from build123d import *
from build123d.topology import SkipClean

# Parameters (mm, degrees)
F_4_40_TAPPED_HOLE1_D               = 2.2606
F_4_40_TAPPED_HOLE1_DEPTH           = 7.62
F_4_40_TAPPED_HOLE1_TIP             = 0.679152758
F_4_40_TAPPED_HOLE1_ON_FACE_2_D     = 2.2606
F_4_40_TAPPED_HOLE1_ON_FACE_2_DEPTH = 7.62
F_4_40_TAPPED_HOLE1_ON_FACE_2_TIP   = 0.679152758
F_4_40_TAPPED_HOLE1_ON_FACE_3_D     = 2.2606
F_4_40_TAPPED_HOLE1_ON_FACE_3_DEPTH = 7.62
F_4_40_TAPPED_HOLE1_ON_FACE_3_TIP   = 0.679152758
F_4_40_TAPPED_HOLE1_ON_FACE_4_D     = 2.2606
F_4_40_TAPPED_HOLE1_ON_FACE_4_DEPTH = 7.62
F_4_40_TAPPED_HOLE1_ON_FACE_4_TIP   = 0.679152758
SKETCH10_R                          = 20.50415
CUT_EXTRUDE3_DEPTH                  = 31.75
F_4_40_TAPPED_HOLE2_D               = 2.2606
F_4_40_TAPPED_HOLE2_DEPTH           = 7.62
F_4_40_TAPPED_HOLE2_TIP             = 0.679152758
CHAMFER1_SIZE                       = 1.27
SKETCH23_R                          = 26.9621
CUT_EXTRUDE6_DEPTH                  = 10
CUT_EXTRUDE7_DEPTH                  = 21.75
FILLET2_R                           = 3.556


# Read off the part's stored shape, not the designer's step: AdvancedHole3
with BuildPart() as part:
    # Sketch2 → Revolve1 (revolve)
    with BuildSketch(Plane(origin=(0, 0, 0), x_dir=(0, 0, -1), z_dir=(1, 0, 0))):
        Polygon((-18.542, 30.02915), (-12.192, 30.02915), (-12.192, 27.9781), (-8.5725, 27.9781), (-8.5725, 30.02915), (-6.0325, 30.02915), (-6.0325, 27.9781), (-2.413, 27.9781), (-2.413, 30.02915), (0, 30.02915), (0, 0), (-18.542, 0), align=None)
    revolve(axis=Axis((0, 0, 0), (0, 0, 1)))

    # #4-40 Tapped Hole1
    with Locations(Plane(origin=(0, -30.02915, 15.367), x_dir=(0, 0, -1), z_dir=(0, -1, 0))):
        with Locations((0, 0)):
            Hole(F_4_40_TAPPED_HOLE1_D / 2, depth=F_4_40_TAPPED_HOLE1_DEPTH)
            with Locations((0, 0, -(F_4_40_TAPPED_HOLE1_DEPTH + F_4_40_TAPPED_HOLE1_TIP / 2))):  # 118° drill point
                Cone(0, F_4_40_TAPPED_HOLE1_D / 2, F_4_40_TAPPED_HOLE1_TIP, mode=Mode.SUBTRACT)

    # #4-40 Tapped Hole1 on face 2
    with Locations(Plane(origin=(30.02915, 0, 15.367), x_dir=(0, 0, 1), z_dir=(1, 0, 0))):
        with Locations((0, 0)):
            Hole(F_4_40_TAPPED_HOLE1_ON_FACE_2_D / 2, depth=F_4_40_TAPPED_HOLE1_ON_FACE_2_DEPTH)
            with Locations((0, 0, -(F_4_40_TAPPED_HOLE1_ON_FACE_2_DEPTH + F_4_40_TAPPED_HOLE1_ON_FACE_2_TIP / 2))):  # 118° drill point
                Cone(0, F_4_40_TAPPED_HOLE1_ON_FACE_2_D / 2, F_4_40_TAPPED_HOLE1_ON_FACE_2_TIP, mode=Mode.SUBTRACT)

    # #4-40 Tapped Hole1 on face 3
    with Locations(Plane(origin=(-30.02915, 0, 15.367), x_dir=(0, 0, -1), z_dir=(-1, 0, 0))):
        with Locations((0, 0)):
            Hole(F_4_40_TAPPED_HOLE1_ON_FACE_3_D / 2, depth=F_4_40_TAPPED_HOLE1_ON_FACE_3_DEPTH)
            with Locations((0, 0, -(F_4_40_TAPPED_HOLE1_ON_FACE_3_DEPTH + F_4_40_TAPPED_HOLE1_ON_FACE_3_TIP / 2))):  # 118° drill point
                Cone(0, F_4_40_TAPPED_HOLE1_ON_FACE_3_D / 2, F_4_40_TAPPED_HOLE1_ON_FACE_3_TIP, mode=Mode.SUBTRACT)

    # #4-40 Tapped Hole1 on face 4
    with Locations(Plane(origin=(0, 30.02915, 15.367), x_dir=(0, 0, 1), z_dir=(0, 1, 0))):
        with Locations((0, 0)):
            Hole(F_4_40_TAPPED_HOLE1_ON_FACE_4_D / 2, depth=F_4_40_TAPPED_HOLE1_ON_FACE_4_DEPTH)
            with Locations((0, 0, -(F_4_40_TAPPED_HOLE1_ON_FACE_4_DEPTH + F_4_40_TAPPED_HOLE1_ON_FACE_4_TIP / 2))):  # 118° drill point
                Cone(0, F_4_40_TAPPED_HOLE1_ON_FACE_4_D / 2, F_4_40_TAPPED_HOLE1_ON_FACE_4_TIP, mode=Mode.SUBTRACT)

    # Sketch6 → Revolve2 (revolve)
    with BuildSketch(Plane(origin=(0, 0, 0), x_dir=(1, 0, 0), z_dir=(0, 1, 0)), mode=Mode.PRIVATE) as revolve2_sk:
        with BuildLine():
            Line((0, -18.542), (31.75, -18.542))
            ThreePointArc((31.75, -18.542), (22.450640303, -40.992640303), (0, -50.292))
            Line((0, -50.292), (0, -18.542))
        make_face()
    revolve(revolve2_sk.sketch.rotate(Axis((0, 0, 18.542), (0, 0, 1)), 90), axis=Axis((0, 0, 18.542), (0, 0, 1)))

    # Sketch10 → Cut-Extrude3 (cut)
    with BuildSketch(Plane(origin=(0, 0, 0), x_dir=(-1, 0, 0), z_dir=(0, 0, -1))):
        with Locations(Location((0, 0, 0), (0, 0, 90))):
            Circle(SKETCH10_R)
    extrude(amount=-CUT_EXTRUDE3_DEPTH, mode=Mode.SUBTRACT)

    # #4-40 Tapped Hole2
    with Locations(Plane(origin=(0, 0, 31.75), x_dir=(-1, 0, 0), z_dir=(0, 0, -1))):
        with Locations((0, 0)):
            Hole(F_4_40_TAPPED_HOLE2_D / 2, depth=F_4_40_TAPPED_HOLE2_DEPTH)
            with Locations((0, 0, -(F_4_40_TAPPED_HOLE2_DEPTH + F_4_40_TAPPED_HOLE2_TIP / 2))):  # 118° drill point
                Cone(0, F_4_40_TAPPED_HOLE2_D / 2, F_4_40_TAPPED_HOLE2_TIP, mode=Mode.SUBTRACT)

    # Chamfer1
    chamfer1_edges = [part.edges().sort_by_distance(p)[0] for p in [
        (0, -30.02915, 0),
    ]]
    chamfer(chamfer1_edges, length=CHAMFER1_SIZE)

    # AdvancedHole3 outline → AdvancedHole3 (revolve, cut)
    with BuildSketch(Plane.YX.offset(-36.83)):
        Polygon((3.81, 28.256858344), (0, 28.256858344), (0, 8.880183098), (2.5527, 10.414), (2.5527, 23.114), (3.81, 23.114), align=None)
    advancedhole3 = revolve(axis=Axis((0, 0, 36.83), (1, 0, 0)), mode=Mode.SUBTRACT)

    # Mirror2: AdvancedHole3 across plane
    add(advancedhole3.mirror(Plane(origin=(0, 0, 0), x_dir=(0, 0, 1), z_dir=(1, 0, 0))), mode=Mode.SUBTRACT)

    # Sketch23 → Cut-Extrude6 (cut)
    with BuildSketch(Plane(origin=(0, 0, 0), x_dir=(-1, 0, 0), z_dir=(0, 0, -1))):
        with Locations(Location((0, 0, 0), (0, 0, 90))):
            Circle(SKETCH23_R)
    extrude(amount=-CUT_EXTRUDE6_DEPTH, mode=Mode.SUBTRACT)

    # Sketch24 → Cut-Extrude7 (cut)
    with SkipClean():  # the faces are left unmerged after this step: merging them gives an invalid solid
        with BuildSketch(Plane(origin=(0, 0, 10), x_dir=(-1, 0, 0), z_dir=(0, 0, -1))):
            with BuildLine():
                Line((-5.972908248, 26.29218902), (-2.54, 20.346217516))
                Line((-2.54, 20.346217516), (2.54, 20.346217516))
                Line((2.54, 20.346217516), (5.972908248, 26.29218902))
                ThreePointArc((5.972908248, 26.29218902), (19.065083745, 19.065083745), (26.29218902, 5.972908248))
                Line((26.29218902, 5.972908248), (20.346217516, 2.54))
                Line((20.346217516, 2.54), (20.346217516, -2.54))
                Line((20.346217516, -2.54), (26.29218902, -5.972908248))
                ThreePointArc((26.29218902, -5.972908248), (19.065083745, -19.065083745), (5.972908248, -26.29218902))
                Line((5.972908248, -26.29218902), (2.54, -20.346217516))
                Line((2.54, -20.346217516), (-2.54, -20.346217516))
                Line((-2.54, -20.346217516), (-5.972908248, -26.29218902))
                ThreePointArc((-5.972908248, -26.29218902), (-19.065083745, -19.065083745), (-26.29218902, -5.972908248))
                Line((-26.29218902, -5.972908248), (-20.346217516, -2.54))
                Line((-20.346217516, -2.54), (-20.346217516, 2.54))
                Line((-20.346217516, 2.54), (-26.29218902, 5.972908248))
                ThreePointArc((-26.29218902, 5.972908248), (-19.065083745, 19.065083745), (-5.972908248, 26.29218902))
            make_face()
        extrude(amount=-CUT_EXTRUDE7_DEPTH, mode=Mode.SUBTRACT)

    # Fillet2
    fillet2_edges = [part.edges().sort_by_distance(p)[0] for p in [
        (26.29218902, 5.972908248, 20.875),
        (5.972908248, 26.29218902, 20.875),
        (-5.972908248, 26.29218902, 20.875),
        (-26.29218902, 5.972908248, 20.875),
        (-26.29218902, -5.972908248, 20.875),
        (-5.972908248, -26.29218902, 20.875),
        (5.972908248, -26.29218902, 20.875),
        (26.29218902, -5.972908248, 20.875),
    ]]
    fillet(fillet2_edges, radius=FILLET2_R)


solid = part.part
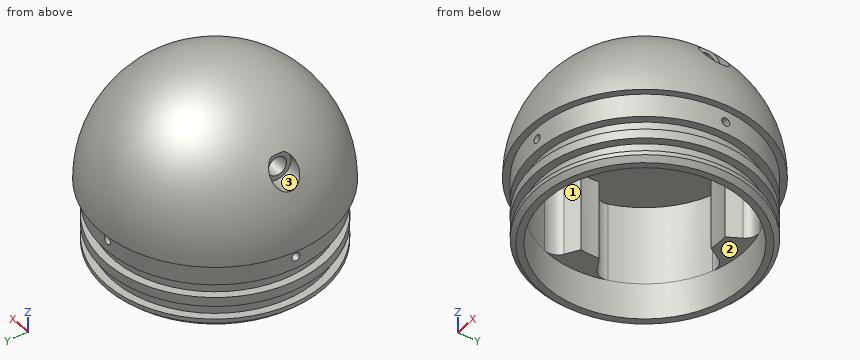
Source: CAD feature listing. Evaluate the final solid. Frame: model axes, mm. Face numbers are marked on the shaded views. Coordinates: 2 decimals unless noted, no trailing zeros. Loops run counter-clockwise (first coordinate to the right, second up) from the corner with the lowest first, then second, coordinate; pieces in that order, holes last. Notation, with made-up numbers: M -38,74.25 L -31,74.25 A31 cw -31,106.25 Z; hole C 17.5,-28.75 d8. An arc over 180 degrees is marked long. Answer in a Markdown table with one row per item.
Q1. Section B-B on z = 41.5. Return the cut outline in (x, y).
Answers below:
| item | result |
|---|---|
| outline | C 0,0 d43.86 |
Q2. Draft query along Z for the marked faces 1, 2 and 3. Return one class per face: pulls with the +Z half, pulls with the -Z half, needs draft (parallel to the pull), parting line crosses it, or undercut.
Answers below:
| item | result |
|---|---|
| face 1 | needs draft |
| face 2 | pulls with the -Z half |
| face 3 | undercut |
Q3. Section A-A on z = 22. Return the cut outline in (x, y), plus the area to 3 significant figures.
Answers below:
| item | result |
|---|---|
| outline | C 0,0 d63.12; hole M -25.47,-8.83 A26.96 ccw -8.83,-25.47 A3.56 ccw -4.59,-23.89 L -2.54,-20.35 A20.5 ccw 2.54,-20.35 L 4.59,-23.89 A3.56 ccw 8.83,-25.47 A26.96 ccw 25.47,-8.83 A3.56 ccw 23.89,-4.59 L 20.35,-2.54 A20.5 ccw 20.35,2.54 L 23.89,4.59 A3.56 ccw 25.47,8.83 A26.96 ccw 8.83,25.47 A3.56 ccw 4.59,23.89 L 2.54,20.35 A20.5 ccw -2.54,20.35 L -4.59,23.89 A3.56 ccw -8.83,25.47 A26.96 ccw -25.47,8.83 A3.56 ccw -23.89,4.59 L -20.35,2.54 A20.5 ccw -20.35,-2.54 L -23.89,-4.59 A3.56 ccw Z |
| area | 1,080 mm^2 |
Q4. Ray query, probe 1 along X at (y, z) = (-0.5, 12.5); probe 2 along Z at (x, y) = (-15, 25); probe 3 along Y at (x, z) = (0, 4). Return the intervals inside material, ascending. Write a range as from..to.
Answers below:
| item | result |
|---|---|
| probe 1 | x = -30.02..-20.5, 20.5..30.02 |
| probe 2 | z = 0.4..2.41, 6.03..8.57, 12.19..31.11 |
| probe 3 | y = -27.98..-26.96, 26.96..27.98 |
Q5. First-contact query: pin 1 (8 mm diameter, centred on y = 1, z = 35.5, fed in from -X); pin 2 (4 mm diameter, centred on x = -21.5, z = 10, fed in from -Y); pin 3 (12 mm diameter, centred on x = 11, z = 9.5, fed in from +Y). Flat tips, straight axial feed; report the tip coordinate or a pass-through.
Answers below:
| item | result |
|---|---|
| pin 1 | stops at x = -28.97 |
| pin 2 | stops at y = -22.31 |
| pin 3 | stops at y = 29.6 |
